Check sheet for the drawn part. Datum: minimum x, y, z corner. Units: mm. Round coordinates to 2 decimals unless told otherwise and drop trailing zeros. Loops run counter-clockwise (first coordinate to the right, second up) from the corner with the lowest first, then second, coordinate; pieces in that order, holes last. Notation, with made-up numbers: (43, -15.5) -> (73, -15.5) arc R20 cw to (73, 18.5) -> close; hole circle Ø3 at (-21.5, 15.5). An arc over 180 degrees is marked (long way). Return JSON: item names as keys, results as strings.
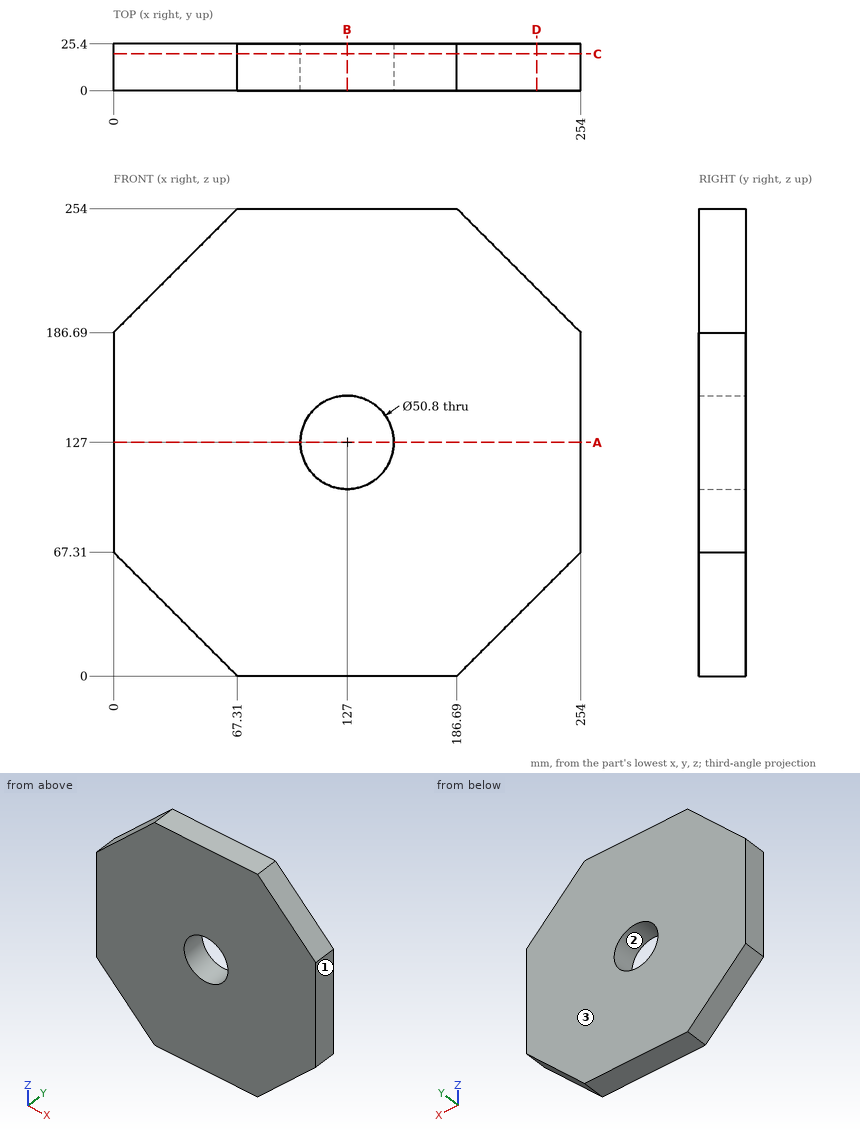
Q1. Draft check along X on the marked faces 1, 2 and 3. Enter one of: released by +X, released by -X, zero draft, split by the parting line, or undercut.
Results list:
{"face 1": "released by +X", "face 2": "undercut", "face 3": "zero draft"}
Q2. Section check A-A (z = 127). Record the boundary of the cut face in (x, y).
Results list:
{"outline": "(0, 0) -> (101.6, 0) -> (101.6, 25.4) -> (0, 25.4) -> close; (152.4, 0) -> (254, 0) -> (254, 25.4) -> (152.4, 25.4) -> close"}
Q3. Section check C-C (y = 20). Record the boundary of the cut face in (x, z).
Results list:
{"outline": "(0, 67.31) -> (67.31, 0) -> (186.69, 0) -> (254, 67.31) -> (254, 186.69) -> (186.69, 254) -> (67.31, 254) -> (0, 186.69) -> close; hole circle Ø50.8 at (127, 127)"}
Q4. Section check D-D (x = 230). Record the boundary of the cut face in (y, z).
Results list:
{"outline": "(0, 43.31) -> (25.4, 43.31) -> (25.4, 210.69) -> (0, 210.69) -> close"}
Q5. Go/stop test with a flat-tipped pin: pin 1 (8 mm diameter, centred on x = 30.5, y = 19.5, fed in from +Z). Record where the tip stops, or that it passes through.
Results list:
{"pin 1": "z = 221.19"}
Q6. Material ranges on line 1 (Z direction, x = 127, y = 9.25); line 2 (Z direction, x = 134, y = 6), recorded low to high.
Results list:
{"line 1": "0 to 101.6, 152.4 to 254", "line 2": "0 to 102.58, 151.42 to 254"}
Q7. Section check B-B (x = 127). Record the boundary of the cut face in (y, z).
Results list:
{"outline": "(0, 0) -> (25.4, 0) -> (25.4, 101.6) -> (0, 101.6) -> close; (0, 152.4) -> (25.4, 152.4) -> (25.4, 254) -> (0, 254) -> close"}
